from build123d import *

# Parameters (mm, degrees)
F1_DEPTH = 38.1
F3_DEPTH = 12.7
F4_DEPTH = 12.7
F6_DEPTH = 12.7


with BuildPart() as f1:
    # F0 (on Front) → F1 (new body)
    with BuildSketch(Plane.XZ):
        Polygon((0, 31.75), (0, 0), (54.61, 0), (44.45, 31.75), align=None)
    extrude(amount=F1_DEPTH)

    # F2 (on face) → F3 (cut)
    with BuildSketch(Plane(origin=(0, 0, 0), x_dir=(-1, 0, 0), z_dir=(0, 1, 0))):
        Polygon((44.420516, 31.673804), (19.705663, 31.673804), (28.255075, -0.054016), (54.679817, -0.054016), align=None)
        Polygon((-44.45, 31.75), (-54.61, 0), (-29.17323, 0), (-19.05, 31.75), align=None)
    extrude(amount=-F3_DEPTH, mode=Mode.SUBTRACT)

    # F2 (on face) → F4 (cut)
    with BuildSketch(Plane(origin=(0, 0, 0), x_dir=(-1, 0, 0), z_dir=(0, 1, 0))):
        Polygon((44.420516, 31.673804), (19.705663, 31.673804), (28.255075, -0.054016), (54.679817, -0.054016), align=None)
        Polygon((-44.45, 31.75), (-54.61, 0), (-29.17323, 0), (-19.05, 31.75), align=None)
    extrude(amount=-F4_DEPTH, mode=Mode.SUBTRACT)

    # F5 (on face) → F6 (cut)
    with BuildSketch(Plane.XZ.offset(38.1)):
        Polygon((29.21, 0), (54.61, 0), (44.45, 31.75), (19.08677, 31.75), align=None)
    extrude(amount=-F6_DEPTH, mode=Mode.SUBTRACT)


solid = f1.part
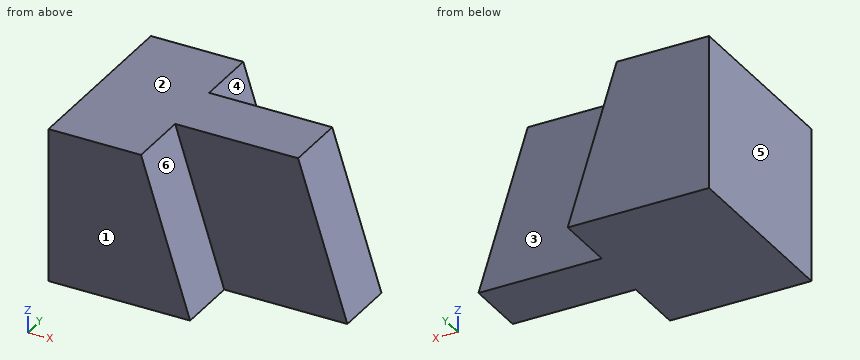
Read the model definition and answer for the solid it produces. Units are mm, in the model's axes. Face numbers are marked on the shaded views. A direction names the side the tool comes from. Give positions to 0.01 mm unless a question says otherwise; leave off trailing zeros. Write each loop counter-clockwise with the first axis right and the second up, starting at its lowest first coordinate (ties: lowest second). Pieces come first, ordered by that corner, then holes. Notation, with made-up numbers: (50.5, 52.5) - (90.5, 52.5) arc R21 cw to (90.5, 71.5) - close; hole circle Ø1 at (29.5, -2.75). An arc over 180 degrees is marked (long way). Use CSV: the item, a comma, the result in double quotes. Start each with the question number.
(1) Find section D-D (z = 22.5). Give the vertices of the cut face in (x, y).
(2) For the marked faces 4, 5 and 6, determine the directions among +Z, -Z, +X, -X, +Y, -Y from which every point of the face is accessible in a straight line to the end or side of a thin tool.
(3) Determine the mould class of the marked faces 1, 2 and 3 for opening direction Y: +Y half, -Y half, draft (parallel to the pull), parting line (faces both ways), or undercut.
(4) Find section A-A (z = 17). Give the vertices of the cut face in (x, y).
(5) Find section C-C (x = 34.5). Give the vertices of the cut face in (y, z).
(6) Given P1, Ø2, axis at x = 42.5, z = 13, coming from the +Y side; P2, Ø4, axis at y = -13.5, z = 7, coming from the +X side, each flat-ended and moving along its own axis, determine where each tip first touches the part or whether it passes through.
(7) Consider line 1 along Y through (x, z) = (34, 22); line 2 along X through (y, z) = (-33.5, 21.5); line 3 along X through (y, z) = (-8, 15.5). Determine where each line is inside the solid, lowest interval first.
(8) Find section B-B (y = -22). Give the vertices of the cut face in (x, z), plus the area to 3 significant figures.
Findings below:
1,outline,"(0, -38.1) - (22.04, -38.1) - (22.04, -25.4) - (47.41, -25.4) - (47.41, -12.7) - (22, -12.7) - (22, 0) - (0, 0) - close"
2,face 4,"+Z, +X, +Y"
2,face 5,"+Z, -Z, -X, +Y, -Y"
2,face 6,"+Z, +X, -Y"
3,face 1,"-Y half"
3,face 2,"draft"
3,face 3,"+Y half"
4,outline,"(0, -38.1) - (23.79, -38.1) - (23.79, -25.4) - (49.17, -25.4) - (49.17, -12.7) - (23.75, -12.7) - (23.75, 0) - (0, 0) - close"
5,outline,"(-25.4, 0) - (-12.7, 0) - (-12.7, 31.75) - (-25.4, 31.75) - close"
6,P1,"y = -12.7"
6,P2,"x = 53.01"
7,line 1,"-25.4 to -12.7"
7,line 2,"0 to 22.35"
7,line 3,"0 to 24.23"
8,outline,"(0, 0) - (54.61, 0) - (44.45, 31.75) - (0, 31.75) - close"
8,area,"1,570 mm2"
